Source: three-view drawing plus pictorial views. Frame: mm from the lowest corner of the part. A direction names the side the tool comes from. Give positions to 0.01 mm unless a question says otherwise; leave off trailing zeros. Loops run counter-clockwise (first coordinate to the right, second up) from the corner with the lowest first, then second, coordinate; pieces in that order, holes last.
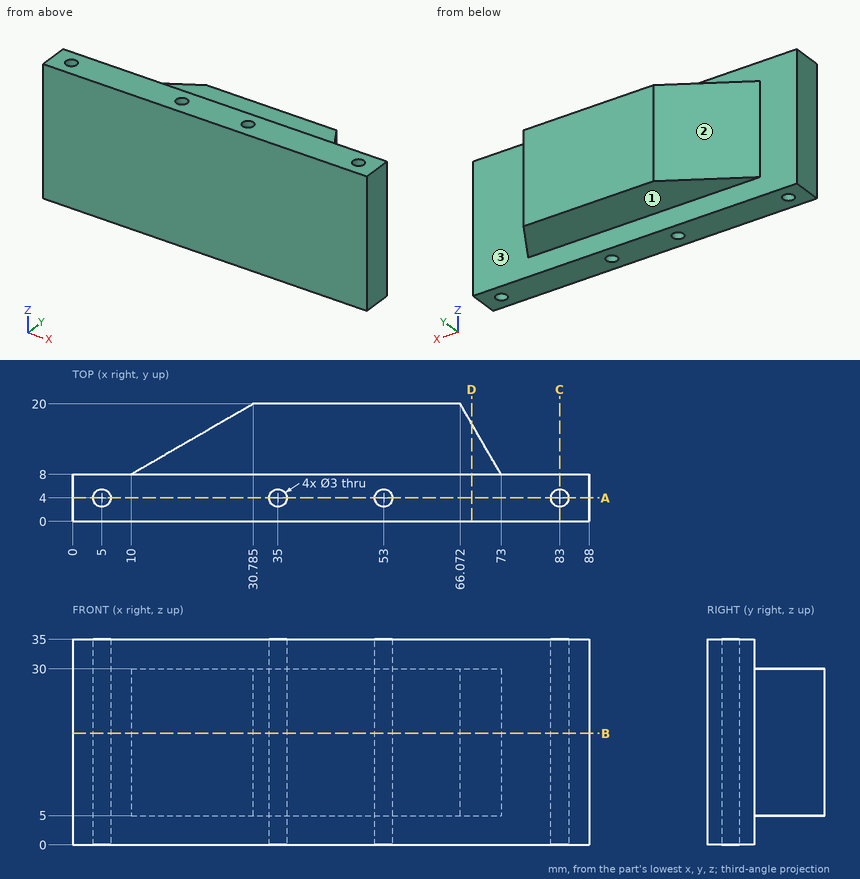
(1) Reachability of the marked faces 1, 2 and 3 from +Z, -Z, +X, -X, +Y, -Y: full face, straight path, thin tool, end or side. Return the list, or none.
Values follow:
face 1: -Z, +X, -X, +Y
face 2: +Z, -Z, -X, +Y
face 3: +Y
(2) Cut plane B-B (z = 19). Return the cut outline in (x, y) (1 decimal).
Values follow:
outline: (0, 0) - (88, 0) - (88, 8) - (73, 8) - (66.1, 20) - (30.8, 20) - (10, 8) - (0, 8) - close; hole circle Ø3 at (5, 4); hole circle Ø3 at (35, 4); hole circle Ø3 at (53, 4); hole circle Ø3 at (83, 4)
(3) Cut plane D-D (x = 68). Return the cut outline in (y, z).
Values follow:
outline: (0, 0) - (8, 0) - (8, 5) - (16.66, 5) - (16.66, 30) - (8, 30) - (8, 35) - (0, 35) - close
(4) Pin query (flat end, axial travel): pin 1 Ø2 at (y, z) = (13.5, 9) entering from +X; pin 2 Ø10 at (x, y) = (27, 14) entering from +Z; pin 3 Ø6 at (y, z) = (16.5, 8) entering from +X (1 decimal). Return the tip coordinate at first contact, or that it passes through.
Values follow:
pin 1: stops at x = 70.4
pin 2: stops at z = 30
pin 3: stops at x = 69.8
(5) Ray query, probe 1 along X at (y, z) = (5.25, 4); probe 2 along Y at (x, z) = (5, 14); probe 3 along Y at (x, z) = (53, 8). Return the intervals inside material, ascending.
Values follow:
probe 1: x = 0 to 4.17, 5.83 to 34.17, 35.83 to 52.17, 53.83 to 82.17, 83.83 to 88
probe 2: y = 0 to 2.5, 5.5 to 8
probe 3: y = 0 to 2.5, 5.5 to 20
(6) Cut plane C-C (x = 83). Return the cut outline in (y, z), and give its area (3 significant figures).
Values follow:
outline: (0, 0) - (2.5, 0) - (2.5, 35) - (0, 35) - close; (5.5, 0) - (8, 0) - (8, 35) - (5.5, 35) - close
area: 175 mm2
(7) Cut plane A-A (y = 4). Return the cut outline in (x, z), and give its area (3 significant figures).
Values follow:
outline: (0, 0) - (3.5, 0) - (3.5, 35) - (0, 35) - close; (6.5, 0) - (33.5, 0) - (33.5, 35) - (6.5, 35) - close; (36.5, 0) - (51.5, 0) - (51.5, 35) - (36.5, 35) - close; (54.5, 0) - (81.5, 0) - (81.5, 35) - (54.5, 35) - close; (84.5, 0) - (88, 0) - (88, 35) - (84.5, 35) - close
area: 2,660 mm2
